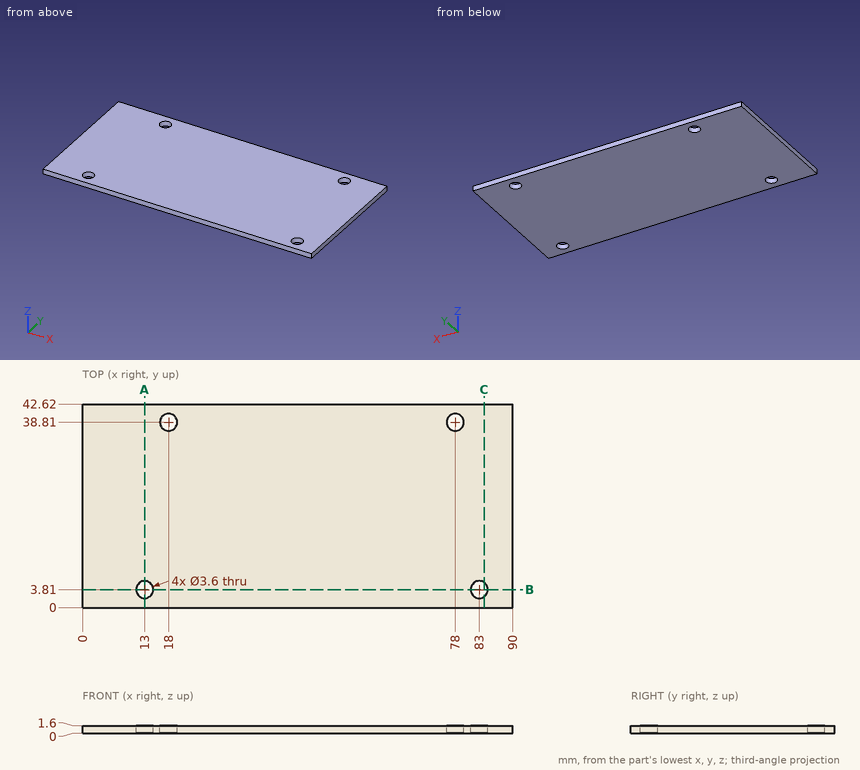
Job drawing, mm, ordinate dimensions from the low corner. One solid piece. Give positions to 0.01 mm unless a question says otherwise; leave off trailing zeros. Loops run counter-clockwise (first coordinate to the right, second up) from the corner with the lowest first, then second, coordinate; pieces in that order, holes last. Notation, with made-up numbers: (50, 18) -> (84, 18) arc R23 cw to (84, 50) -> close; hole circle Ø10 at (40, 56). An arc over 180 degrees is marked (long way). Write each question's results on one line, items separated by ' | '. Start each with the question number.
Q1. Wall check: L1, parallel to X at y = 38.81, z = 0.65; L2, parallel to Y at x = 13, z = 0.85; L3, parallel to Y at x = 78, z = 0.8. Give the ranges that are in metal, low to high.
Q2. Band-saw the part on A-A on x = 13. List the corners of the cut face in (y, z), plus the area to 3 significant figures.
Q3. Band-saw the part on B-B on y = 3.81. List the corners of the cut face in (x, z).
Q4. Pin check, flat tip, straight feed: P1, Ø3, axis at x = 13, y = 3.81, coming from the +Z side. Stop position of the tip, or through.
Q5. Band-saw the part on C-C on x = 84. List the corners of the cut face in (y, z), plus the area to 3 significant figures.
Results are:
1) L1: x = 0 to 16.2, 19.8 to 76.2, 79.8 to 90 | L2: y = 0 to 2.01, 5.61 to 42.62 | L3: y = 0 to 37.01, 40.61 to 42.62
2) outline: (0, 0) -> (2.01, 0) -> (2.01, 1.6) -> (0, 1.6) -> close; (5.61, 0) -> (42.62, 0) -> (42.62, 1.6) -> (5.61, 1.6) -> close | area: 62.4 mm²
3) outline: (0, 0) -> (11.2, 0) -> (11.2, 1.6) -> (0, 1.6) -> close; (14.8, 0) -> (81.2, 0) -> (81.2, 1.6) -> (14.8, 1.6) -> close; (84.8, 0) -> (90, 0) -> (90, 1.6) -> (84.8, 1.6) -> close
4) P1: passes through
5) outline: (0, 0) -> (2.31, 0) -> (2.31, 1.6) -> (0, 1.6) -> close; (5.31, 0) -> (42.62, 0) -> (42.62, 1.6) -> (5.31, 1.6) -> close | area: 63.4 mm²
